Drawing for the job (mm, zero at the part's lowest x, y, z). A direction names the side the tool comes from. Coordinates: 2 decimals unless noted, no trailing zeros. Order: outer loops, then holes, each group sorted by start corner. A loop starts at its lowest first (then second) coordinate and runs counter-clockwise, first axis right, second up.
1) Cut at C-C (x = 2.25). List the corners of the cut face in (y, z).
2) Mould opens along X. For the marked faces 1, 2, 3 and 4 say: +X half, -X half, draft (parallel to the pull), parting line (faces both ways), or undercut.
3) Tool access for the marked faces 5, 6 and 7: list every direction of +Z, -Z, +X, -X, +Y, -Y with a clear straight run to the whole face (end or side of a thin tool).
4) Wall check: L1, parallel to Y at x = 1.8, z = 2.7; L2, parallel to Y at x = 0.7, z = 2.85; L3, parallel to X at y = 10.75, z = 2.5 (1 decimal). Give the ranges that are in metal, low to high.
5) Pin check, flat tip, straight feed: pin 1 Ø0.8 at (x, z) = (1.5, 1.5) entering from +Y. Stop position of the tip, or through.
6) Cut at A-A (y = 9). List the corners of the cut face in (x, z).
7) Cut at D-D (y = 1.25). List the corners of the cut face in (x, z).
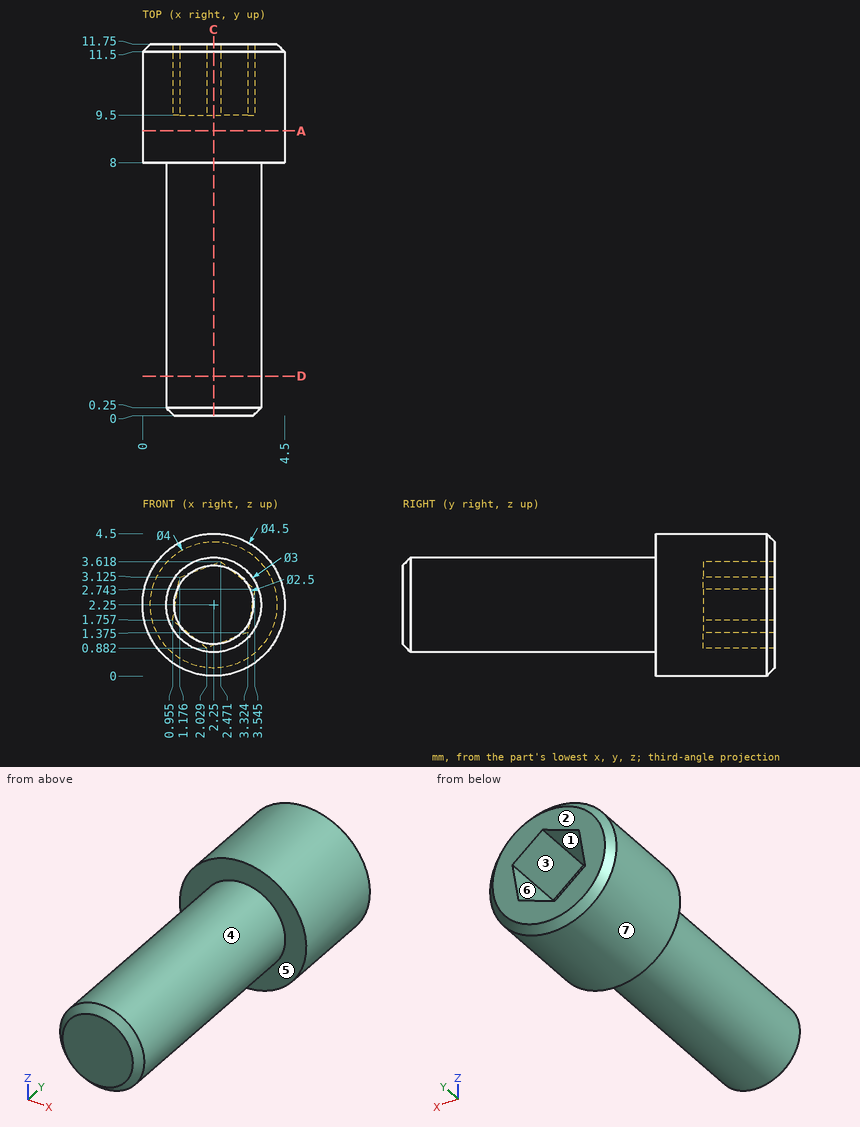
Geometry check:
1. outline: (0, 1) - (0.25, 0.75) - (8, 0.75) - (8, 0) - (11.5, 0) - (11.75, 0.25) - (11.75, 0.97) - (9.5, 0.97) - (9.5, 3.53) - (11.75, 3.53) - (11.75, 4.25) - (11.5, 4.5) - (8, 4.5) - (8, 3.75) - (0.25, 3.75) - (0, 3.5) - close
2. face 1: undercut
2. face 2: draft
2. face 3: undercut
2. face 4: parting line
3. face 5: -Y
3. face 6: +Y
3. face 7: +Y, -Y
4. L1: y = 0 to 9.5
4. L2: y = 8 to 11.75
4. L3: x = 0 to 1.1, 3.5 to 4.5
5. pin 1: stops at y = 11.75
6. outline: circle Ø4.5 at (2.25, 2.25)
7. outline: circle Ø3 at (2.25, 2.25)
